Input: part model. Units: mm. Frame: model coordinates. Give positions to 0.01 mm unless a question says otherwise; leave off trailing zeros. Loops run counter-clockwise (first coordinate to the right, second up) from the corner with the lowest first, then second, coordinate; pieces in that order, holes last.
from build123d import *

# Parameters (mm, degrees)
BOSS_EXTRUDE1_DEPTH     = 3.175
SKETCH4_W               = 38.1
SKETCH4_H               = 152.4
CUT_EXTRUDE2_DEPTH      = 1
CUT_EXTRUDE2_DEPTH_BACK = 4.175
SKETCH2_W               = 177.8
SKETCH2_H               = 254
CUT_EXTRUDE1_DEPTH      = 1
CUT_EXTRUDE1_DEPTH_BACK = 4.175


with BuildPart() as part:
    # Sketch1 → Boss-Extrude1 (new body)
    with BuildSketch(Plane(origin=(0, 0, 0), x_dir=(1, 0, 0), z_dir=(0, 1, 0))):
        Polygon((-139.7, 0), (0, 0), (0, 161.925), (-12.7, 161.925), (-12.7, 165.1), (-38.1, 165.1), (-38.1, 161.925), (-63.5, 161.925), (-63.5, 165.1), (-88.9, 165.1), (-88.9, 161.925), (-114.3, 161.925), (-114.3, 165.1), (-139.7, 165.1), (-139.7, 139.7), (-136.525, 139.7), (-136.525, 114.3), (-139.7, 114.3), (-139.7, 88.9), (-136.525, 88.9), (-136.525, 63.5), (-139.7, 63.5), (-139.7, 38.1), (-136.525, 38.1), (-136.525, 12.7), (-139.7, 12.7), align=None)
    extrude(amount=BOSS_EXTRUDE1_DEPTH)

    # Mirror1: part across plane


with BuildPart() as part_1:
    add(part.part)
    add(part.part.mirror(Plane(origin=(-139.7, 3.175, 0), x_dir=(1, 0, 0), z_dir=(0, 0, -1))))

    # Sketch4 → Cut-Extrude2 (cut, two sides)
    with BuildSketch(Plane(origin=(0, 3.175, 0), x_dir=(1, 0, 0), z_dir=(0, 1, 0))) as cut_extrude2_sk:
        with Locations((-120.65, 78.9)):
            Rectangle(SKETCH4_W, SKETCH4_H)
    extrude(amount=CUT_EXTRUDE2_DEPTH, mode=Mode.SUBTRACT)
    extrude(cut_extrude2_sk.sketch, amount=-CUT_EXTRUDE2_DEPTH_BACK, mode=Mode.SUBTRACT)

    # Mirror2: part across plane


with BuildPart() as part_2:
    add(part_1.part)
    add(part_1.part.mirror(Plane(origin=(0, 3.175, 0), x_dir=(0, 0, 1), z_dir=(-1, 0, 0))))

    # Sketch2 → Cut-Extrude1 (cut, two sides)
    with BuildSketch(Plane(origin=(0, 3.175, 0), x_dir=(1, 0, 0), z_dir=(0, 1, 0))) as cut_extrude1_sk:
        Rectangle(SKETCH2_W, SKETCH2_H)
    extrude(amount=CUT_EXTRUDE1_DEPTH, mode=Mode.SUBTRACT)
    extrude(cut_extrude1_sk.sketch, amount=-CUT_EXTRUDE1_DEPTH_BACK, mode=Mode.SUBTRACT)


solid = part_2.part
(1) Ray query, probe 1 along X at (y, z) = (1.3, -40); probe 2 along X at (y, z) = (0.25, 70) (3 decimals); probe 3 along Z at (x, y) = (8.5, 0.3) (3 decimals). Return the intervals inside material, ascending.
Values follow:
probe 1: x = -101.6 to -88.9, 88.9 to 101.6
probe 2: x = -136.525 to -88.9, 88.9 to 136.525
probe 3: z = -161.925 to -127, 127 to 161.925
(2) Cut plane C-C (z = -142). Return the cut outline in (x, y) (3 decimals).
Values follow:
outline: (-101.6, 0) - (101.6, 0) - (101.6, 3.175) - (-101.6, 3.175) - close
(3) Cut plane B-B (z = -13.5). Return the cut outline in (x, y) (3 decimals).
Values follow:
outline: (-101.6, 0) - (-88.9, 0) - (-88.9, 3.175) - (-101.6, 3.175) - close; (88.9, 0) - (101.6, 0) - (101.6, 3.175) - (88.9, 3.175) - close
(4) Cut plane A-A (x = -81.5). Return the cut outline in (y, z) (3 decimals).
Values follow:
outline: (0, -165.1) - (3.175, -165.1) - (3.175, -127) - (0, -127) - close; (0, 127) - (3.175, 127) - (3.175, 165.1) - (0, 165.1) - close
(5) Pin query (flat end, axial travel): pin 1 Ø1 at (x, y) = (-45, 2.5) entering from +Z (3 decimals); pin 2 Ø1 at (x, y) = (52.5, 1.5) entering from -Z (3 decimals); pin 3 Ø1.6 at (y, z) = (1.5, 130) entering from -X (3 decimals). Return the tip coordinate at first contact, or that it passes through.
Values follow:
pin 1: stops at z = 161.925
pin 2: stops at z = -161.925
pin 3: stops at x = -136.525
